Model file for the job. Use its own axes, mm. A direction names the side the tool comes from. Round coordinates to 2 decimals unless told otherwise and drop trailing zeros. Order: outer loops, then holes, each group sorted by start corner. A loop starts at its lowest first (then second) coordinate and runs counter-clockwise, first axis right, second up. Notation, with made-up numbers: (52.5, 80.5) - (98.5, 80.5) arc R23 ccw to (98.5, 114.5) - close; hole circle Ø7 at (79, 89.25). An arc over 180 degrees is marked (long way). Use one line per item in the form item = value.
Autodesk Inventor part; units mm, degrees
ref_plane "YZ Plane" through (0, 0, 0) normal (1, 0, 0) x (0, 1, 0)
ref_plane "XZ Plane" through (0, 0, 0) normal (0, 1, 0) x (-1, 0, 0)
ref_plane "XY Plane" through (0, 0, 0) normal (0, 0, 1) x (1, 0, 0)
sketch "Sketch1" plane through (0, 0, 0) normal (0, 0, 1) x (1, 0, 0)
  circle A0 centre (0, 0) radius 7.5
  line L0 (2, -2.25) -> (2, -10.25)
  line L1 (2, -10.25) -> (-2, -10.25)
  line L2 (-2, -10.25) -> (-2, -2.25)
  point P0 (0, 0)
  point P1 (0, 0)
  point P2 (-2, -7.2284)
  point P3 (2, -7.2284)
extrude "Extrusion1" add sketch "Sketch1" along normal blind 3
fillet "Fillet1" radius 2 2 edges at (2, -10.25, 1.5) (-2, -10.25, 1.5)
mirror "Mirror1" about plane through (0, 0, 0) normal (0, 1, 0)
properties part number "try"
(1) Slice it at B-B on y = -8. Give the cut face in (x, z), then the cut area to 3 significant figures.
Report:
outline = (-2, 0) - (2, 0) - (2, 3) - (-2, 3) - close
area = 12.0 mm2
(2) Slice it at C-C on x = -6. Give the cut face in (y, z), then the cut area to 3 significant figures.
Report:
outline = (-4.5, 0) - (4.5, 0) - (4.5, 3) - (-4.5, 3) - close
area = 27.0 mm2
(3) Tool access for faces 1 (the face through (2, -8, 1)), 2 (the face through (-2, -8, 1)), 3 (the face through (2, 8, 1)), 4 (the face through (-2, 8, 1)): list every direction of +Z, -Z, +X, -X, +Y, -Y with a clear straight run to the whole face (end or side of a thin tool).
Report:
face_1 = +Z, -Z, +X, -Y
face_2 = +Z, -Z, -X, -Y
face_3 = +Z, -Z, +X, +Y
face_4 = +Z, -Z, -X, +Y
(4) Probe probe 1 along Y at (x, z) = (-1, 2); probe 2 along Y at (x, z) = (-3, 1.55); probe 3 along X at (y, z) = (-1.5, 0.3). List the from-to ranges inside material, lowest first. Write a range as [from, to].
Report:
probe_1 = [-9.98, 9.98]
probe_2 = [-6.87, 6.87]
probe_3 = [-7.35, 7.35]
(5) Pin check, flat tips, straight feed: pin 1 (1.1 mm diameter, centred on y = 7.5, z = 1.5, fed in from -X); pin 2 (1.5 mm diameter, centred on x = 2, z = 1.5, fed in from +Y); pin 3 (1.1 mm diameter, centred on y = -8, z = 1, fed in from +X). Stop position of each tip, or through.
Report:
pin_1 = -2.82
pin_2 = 9.81
pin_3 = 2
